Read the model definition and answer for the solid it produces. Units are mm, in the model's axes. A direction names the side the tool comes from. Coordinates: 2 decimals unless noted, no trailing zeros. Write each loop counter-clockwise with the first axis right and the second up, starting at its lowest first coordinate (ties: lowest second). Pieces come first, ordered by that corner, then holes. Notation, with made-up numbers: (-15.75, 41.5) -> (37.25, 41.5) arc R13 ccw to (37.25, 58.5) -> close; hole circle Ø8 at (-12.5, 38). An arc over 180 degrees is marked (long way). One line per item, written item: value. Start each with the question number.
from build123d import *

# Parameters (mm, degrees)
F0_R          = 19.05
F1_DEPTH      = 63.5
F2_R          = 5.5626
F3_DEPTH      = 4.7752
F3_DEPTH_BACK = 15.875
F5_DEPTH      = 57.151


with BuildPart() as f1:
    # F0 (on Front) → F1 (new body)
    with BuildSketch(Plane.XZ):
        with BuildLine():
            Line((69.85, 28.575), (0, 28.575))
            ThreePointArc((0, 28.575), (-19.345366, -21.030631), (28.475608, 2.38125))
            ThreePointArc((28.475608, 2.38125), (30.957268, 9.623455), (37.967478, 12.7))
            Line((37.967478, 12.7), (69.85, 12.7))
            Line((69.85, 12.7), (69.85, 28.575))
        make_face()
        Circle(F0_R, mode=Mode.SUBTRACT)
    extrude(amount=F1_DEPTH)

    # F2 (on face) → F3 (join, two sides)
    with BuildSketch(Plane.XY.offset(28.575)) as f3_sk:
        with BuildLine():
            ThreePointArc((76.149155, -1.672279), (63.474628, -1.716165), (57.15, -12.7))
            Line((57.15, -12.7), (57.15, -50.8))
            ThreePointArc((57.15, -50.8), (63.474628, -61.783835), (76.149155, -61.827721))
            Line((76.149155, -61.827721), (109.499355, -42.777721))
            ThreePointArc((109.499355, -42.777721), (115.9002, -31.75), (109.499355, -20.722279))
            Line((109.499355, -20.722279), (76.149155, -1.672279))
        make_face()
        with Locations((69.85, -50.8)):
            Circle(F2_R, mode=Mode.SUBTRACT)
        with Locations((69.85, -12.7)):
            Circle(F2_R, mode=Mode.SUBTRACT)
        with Locations((103.2002, -31.75)):
            Circle(F2_R, mode=Mode.SUBTRACT)
    extrude(amount=F3_DEPTH)
    extrude(f3_sk.sketch, amount=-F3_DEPTH_BACK)

    # F4 (on face) → F5 (cut, through all)
    with BuildSketch(Plane.XY.offset(28.575)):
        with BuildLine():
            Line((69.85, -18.2626), (69.85, -7.1374))
            ThreePointArc((69.85, -7.1374), (64.2874, -12.7), (69.85, -18.2626))
        make_face()
        with BuildLine():
            Line((69.85, -56.3626), (69.85, -45.2374))
            ThreePointArc((69.85, -45.2374), (64.2874, -50.8), (69.85, -56.3626))
        make_face()
    extrude(amount=-F5_DEPTH, mode=Mode.SUBTRACT)


solid = f1.part
1. A cutting plane is placed at D-D on x = 2.5. Give the vertices of the cut face in (y, z) (3 decimals), then the cut area to 3 significant figures.
2. A cutting plane is placed at C-C on z = 22. Give the vertices of the cut face in (x, y).
3. Find the intervals of material crossed by probe 1 along Y at (x, z) = (69.85, 28); probe 2 along Z at (x, y) = (0, -29.5) (3 decimals); probe 3 along Z at (x, y) = (62.5, -34.5), in increasing order. Write a range as from..to.
4. A tool of negligible diameter and unlimited length cuts with its end or side. For faces 4 (the face through (68, -31, 12.7)), 5 (the face through (75.156, -11.029, 23.17)), 6 (the face through (68.884, -63.463, 30.053)), 7 (the face through (57.15, -31, 31)), 8 (the face through (69.255, -0.014, 30.053)), from which of +Z, -Z, +X, -X, +Y, -Y can it reach the whole face along a straight path? Write none if from no direction.
5. A cutting plane is placed at B-B on z = 0. Give the vertices of the cut face in (x, y) (3 decimals).
6. Given pin 1 (2.5 mm diameter, centred on y = -29.5, z = 30, fed in from -X); pin 2 (8 mm diameter, centred on x = 81.5, y = -54.5, fed in from -Z); pin 3 (12 mm diameter, centred on x = 50.5, y = -24.5, fed in from +Z) (3 decimals); pin 4 (9 mm diameter, centred on x = 103.2, y = -31.75, fed in from -Z), each flat-ended and moving along its own axis, determine where each tip first touches the part or whether it passes through.
7. A cutting plane is placed at A-A on y = -54. Give the vertices of the cut face in (x, z) (3 decimals).
8. For a pull along X with two mould halves and no side action, classify faces 1 (the face through (93.06, -11.33, 23.17)), 2 (the face through (20, -63.5, 7)), 3 (the face through (98.786, -35.135, 22.881)) as +X half, -X half, draft (parallel to the pull), parting line (faces both ways), or undercut.
Derived:
1. outline: (-63.5, -28.465) -> (0, -28.465) -> (0, -18.885) -> (-63.5, -18.885) -> close; (-63.5, 18.885) -> (0, 18.885) -> (0, 28.575) -> (-63.5, 28.575) -> close
1. area: 1,220 mm2
2. outline: (-18.24, -63.5) -> (69.85, -63.5) arc R12.7 ccw to (76.15, -61.83) -> (109.5, -42.78) arc R12.7 ccw to (109.5, -20.72) -> (76.15, -1.67) arc R12.7 ccw to (69.85, 0) -> (-18.24, 0) -> close; hole circle Ø11.13 at (69.85, -50.8); hole circle Ø11.13 at (69.85, -12.7); hole circle Ø11.13 at (103.2, -31.75)
3. probe 1: y = -63.5..-56.36, -45.24..-18.26, -7.14..0
3. probe 2: z = -28.575..-19.05, 19.05..28.575
3. probe 3: z = 12.7..33.35
4. face 4: -Z, +X, +Y, -Y
4. face 5: +Z, -Z
4. face 6: +Z, -Y
4. face 7: +Z, -X, +Y, -Y
4. face 8: +Z, +Y
5. outline: (-28.575, -63.5) -> (-19.05, -63.5) -> (-19.05, 0) -> (-28.575, 0) -> close; (19.05, -63.5) -> (28.575, -63.5) -> (28.575, 0) -> (19.05, 0) -> close
6. pin 1: stops at x = 57.15
6. pin 2: stops at z = 12.7
6. pin 3: stops at z = 28.575
6. pin 4: passes through
7. outline: (0, 28.575) arc R28.575 ccw (long way) to (28.476, 2.381) arc R9.525 cw to (37.967, 12.7) -> (65.3, 12.7) -> (65.3, 33.35) -> (57.56, 33.35) -> (57.56, 28.575) -> close; (74.4, 12.7) -> (89.853, 12.7) -> (89.853, 33.35) -> (74.4, 33.35) -> close; hole circle Ø38.1 at (0, 0)
8. face 1: +X half
8. face 2: draft
8. face 3: undercut
